Geometry check sheet. Reference: the model listing, model coordinates, mm. Face numbers are marked on the shaded views. A direction names the side the tool comes from. Round coordinates to 2 decimals unless told otherwise and drop trailing zeros. Write each loop counter-clockwise with the first axis right and the second up, starting at its lowest first coordinate (ties: lowest second). Pieces come first, ordered by that corner, then holes.
Item 1: Depth check by flat-ended pin: P1, Ø10, axis at x = 13, z = 20.5, coming from the +Y side; P2, Ø1.5, axis at y = 5.5, z = 22.5, coming from the +X side; P3, Ø2, axis at x = 17.5, y = -0.5, coming from the -Z side. Enter the tip coordinate at first touch or a pass-through.
Item 2: Cross-section at A-A (x = 62.5). Enter the section's corners in (y, z), then the cut area to 3 significant figures.
Item 3: Scan lines: probe 1 along X at (y, z) = (10.5, 6.5); probe 2 along X at (y, z) = (0.7, 24.45); probe 3 along Y at (x, z) = (57, 3). Record each from-to range of solid material in increasing order.
Item 4: Draft check along X on the marked faces 4, 5 and 6. Enter one of: pulls with the +X half, pulls with the -X half, needs draft (parallel to the pull), parting line crosses it, or undercut.
Item 5: Cross-section at C-C (z = 1). Enter the section's corners in (x, y), then the cut area to 3 significant figures.
Item 6: Access from +Z, -Z, +X, -X, +Y, -Y to the whole of each face (thin tool, end or side, straight path). Record for the marked faces 1, 2 and 3.
Item 7: Cross-section at D-D (x = -49.5). Enter the section's corners in (y, z), then the cut area to 3 significant figures.
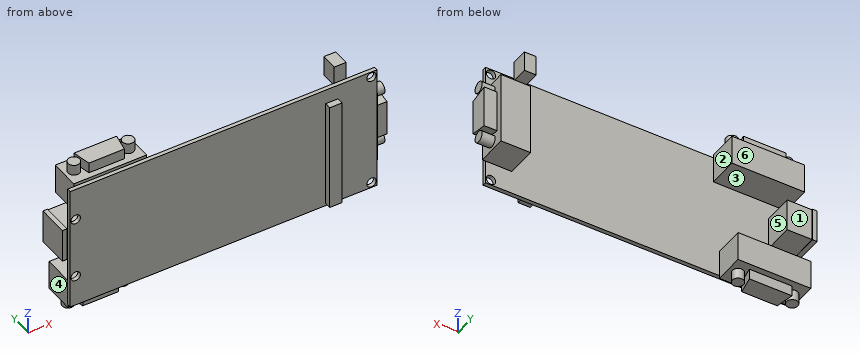
from build123d import *

# Parameters (mm, degrees)
SKETCH1_W           = 129.7
SKETCH1_H           = 53.6
BOARDBASE_DEPTH     = 1.67
SKETCH3_W           = 12.5
SKETCH3_H           = 30.8
BOSS_EXTRUDE2_DEPTH = 12.6
SKETCH4_R           = 2.4
BOSS_EXTRUDE3_DEPTH = 5.5
SKETCH6_W           = 30.8
SKETCH6_H           = 12.5
BOSS_EXTRUDE5_DEPTH = 12.5
SKETCH7_R           = 2.45
BOSS_EXTRUDE6_DEPTH = 4.5
SKETCH5_W           = 30.8
SKETCH5_H           = 12.5
BOSS_EXTRUDE4_DEPTH = 12.6
SKETCH9_R           = 2.4
BOSS_EXTRUDE7_DEPTH = 4.5
SKETCH10_W          = 10.6
SKETCH10_H          = 13.8
BOSS_EXTRUDE8_DEPTH = 12.7
SKETCH12_W          = 14.2
SKETCH12_H          = 13.1
BOSS_EXTRUDE9_DEPTH = 1.9
SKETCH13_W          = 5.2
SKETCH13_H          = 46.3
MOLEXHEADER_DEPTH   = 2.7
SKETCH14_R          = 2
MOUNTHOLES_DEPTH    = 80.767740973
SKETCH15_W          = 5
SKETCH15_H          = 8.5
STIMHEADER_DEPTH    = 7


with BuildPart() as part:
    # Sketch1 → BoardBase (new body)
    with BuildSketch(Plane(origin=(0, 0, 0), x_dir=(1, 0, 0), z_dir=(0, 1, 0))):
        Rectangle(SKETCH1_W, SKETCH1_H)
    extrude(amount=BOARDBASE_DEPTH)

    # Sketch3 → Boss-Extrude2 (add)
    with BuildSketch(Plane(origin=(0, 1.67, 0), x_dir=(1, 0, 0), z_dir=(0, 1, 0))):
        with Locations((59.9, 1.35)):
            Rectangle(SKETCH3_W, SKETCH3_H)
    extrude(amount=BOSS_EXTRUDE2_DEPTH)

    # Sketch4 → Boss-Extrude3 (add)
    with BuildSketch(Plane(origin=(66.15, 0, 0), x_dir=(0, 0, -1), z_dir=(1, 0, 0))):
        with Locations(Location((-10.1, 7.97, 0), (0, 0, 180))):
            Circle(SKETCH4_R)
        with Locations(Location((12.8, 7.97, 0), (0, 0, 180))):
            Circle(SKETCH4_R)
        Polygon((-7.65, 11.77), (10.35, 11.77), (8.85, 4.17), (-6.15, 4.17), align=None)
    extrude(amount=BOSS_EXTRUDE3_DEPTH)

    # Sketch6 → Boss-Extrude5 (add)
    with BuildSketch(Plane(origin=(0, 1.67, 0), x_dir=(1, 0, 0), z_dir=(0, 1, 0))):
        with Locations((-46.9, -21.85)):
            Rectangle(SKETCH6_W, SKETCH6_H)
    extrude(amount=BOSS_EXTRUDE5_DEPTH)

    # Sketch7 → Boss-Extrude6 (add)
    with BuildSketch(Plane.XY.offset(28.1)):
        with Locations(Location((-58.35, 7.92, 0), (0, 0, 180))):
            Circle(SKETCH7_R)
        with Locations(Location((-35.45, 7.92, 0), (0, 0, 180))):
            Circle(SKETCH7_R)
        Polygon((-55.9, 11.72), (-37.9, 11.72), (-39.4, 4.12), (-54.4, 4.12), align=None)
    extrude(amount=BOSS_EXTRUDE6_DEPTH)

    # Sketch5 → Boss-Extrude4 (add)
    with BuildSketch(Plane(origin=(0, 1.67, 0), x_dir=(1, 0, 0), z_dir=(0, 1, 0))):
        with Locations((-49.44, 21.85)):
            Rectangle(SKETCH5_W, SKETCH5_H)
    extrude(amount=BOSS_EXTRUDE4_DEPTH)

    # Sketch9 → Boss-Extrude7 (add)
    with BuildSketch(Plane(origin=(0, 0, -28.1), x_dir=(-1, 0, 0), z_dir=(0, 0, -1))):
        with Locations(Location((37.99, 7.97, 0), (0, 0, 180))):
            Circle(SKETCH9_R)
        with Locations(Location((60.89, 7.97, 0), (0, 0, 180))):
            Circle(SKETCH9_R)
        Polygon((40.44, 11.77), (58.44, 11.77), (56.94, 4.17), (41.94, 4.17), align=None)
    extrude(amount=BOSS_EXTRUDE7_DEPTH)

    # Sketch10 → Boss-Extrude8 (add)
    with BuildSketch(Plane(origin=(0, 1.67, 0), x_dir=(1, 0, 0), z_dir=(0, 1, 0))):
        with Locations((-60.05, -1.6)):
            Rectangle(SKETCH10_W, SKETCH10_H)
    extrude(amount=BOSS_EXTRUDE8_DEPTH)

    # Sketch12 → Boss-Extrude9 (add)
    with BuildSketch(Plane.ZY.offset(65.35)):
        with Locations((1.6, 8.02)):
            Rectangle(SKETCH12_W, SKETCH12_H)
    extrude(amount=BOSS_EXTRUDE9_DEPTH)

    # Sketch13 → MolexHeader (add)
    with BuildSketch(Plane.XZ):
        with Locations((45.75, -2.65)):
            Rectangle(SKETCH13_W, SKETCH13_H)
    extrude(amount=MOLEXHEADER_DEPTH)

    # Sketch14 → MountHoles (cut, through all)
    with BuildSketch(Plane(origin=(0, 1.67, 0), x_dir=(1, 0, 0), z_dir=(0, 1, 0))):
        with Locations(Location((62.5, 24.5, 0), (0, 0, 270))):
            Circle(SKETCH14_R)
        with Locations(Location((62.5, -24.45, 0), (0, 0, 270))):
            Circle(SKETCH14_R)
        with Locations(Location((-62.55, -12.9, 0), (0, 0, 270))):
            Circle(SKETCH14_R)
        with Locations(Location((-62.55, 13.5, 0), (0, 0, 270))):
            Circle(SKETCH14_R)
    extrude(amount=-MOUNTHOLES_DEPTH, mode=Mode.SUBTRACT)

    # Sketch15 → StimHeader (add)
    with BuildSketch(Plane(origin=(0, 1.67, 0), x_dir=(1, 0, 0), z_dir=(0, 1, 0))):
        with Locations((50.25, -30.05)):
            Rectangle(SKETCH15_W, SKETCH15_H)
    extrude(amount=STIMHEADER_DEPTH)


solid = part.part
Resolved:
1. P1: stops at y = 1.67
1. P2: stops at x = -31.5
1. P3: stops at z = -26.8
2. outline: (0, -26.8) - (1.67, -26.8) - (1.67, -26.5) - (0, -26.5) - close; (0, -22.5) - (1.67, -22.5) - (1.67, -16.75) - (14.27, -16.75) - (14.27, 14.05) - (1.67, 14.05) - (1.67, 22.45) - (0, 22.45) - close; (0, 26.45) - (1.67, 26.45) - (1.67, 26.8) - (0, 26.8) - close
2. area: 464 mm2
3. probe 1: x = -67.25 to -54.75, 53.65 to 71.65
3. probe 2: x = -64.85 to 60.5, 64.5 to 64.85
3. probe 3: y = 0 to 14.27
4. face 4: pulls with the -X half
4. face 5: undercut
4. face 6: needs draft
5. outline: (-67.25, 1.47) - (-65.35, 1.47) - (-65.35, 1.67) - (-64.85, 1.67) - (-64.85, 0) - (43.15, 0) - (43.15, -2.7) - (48.35, -2.7) - (48.35, 0) - (64.85, 0) - (64.85, 1.67) - (66.15, 1.67) - (66.15, 4.17) - (71.65, 4.17) - (71.65, 11.77) - (66.15, 11.77) - (66.15, 14.27) - (53.65, 14.27) - (53.65, 1.67) - (-54.75, 1.67) - (-54.75, 14.37) - (-65.35, 14.37) - (-65.35, 14.57) - (-67.25, 14.57) - close
5. area: 589 mm2
6. face 1: +Z, -Z, +X, +Y
6. face 2: +Z, -Z, +Y
6. face 3: +X, -X, +Y
7. outline: (0, -26.8) - (1.67, -26.8) - (1.67, -28.1) - (4.17, -28.1) - (4.17, -32.6) - (11.77, -32.6) - (11.77, -28.1) - (14.27, -28.1) - (14.27, -15.6) - (1.67, -15.6) - (1.67, 15.6) - (14.17, 15.6) - (14.17, 28.1) - (11.72, 28.1) - (11.72, 32.6) - (4.12, 32.6) - (4.12, 28.1) - (1.67, 28.1) - (1.67, 26.8) - (0, 26.8) - close
7. area: 472 mm2
